Could you check a few things on this model? Use its own coordinates, in mm. A direction names the side the tool comes from. Give positions to 0.01 mm unless a question says otherwise; leave off trailing zeros. Loops run counter-clockwise (first coordinate to the right, second up) from the corner with the lowest first, then second, coordinate; pieces in that order, holes last. Notation, with made-up numbers: M 66.25,21.5 L 102.25,21.5 A19 ccw 102.25,43.5 Z; hole C 24.25,-11.5 d1. An arc over 180 degrees is marked long. Answer in a Markdown table with one row per item. Add a question column.
```python
from build123d import *

# Parameters (mm, degrees)
SKETCH1_R                = 14.5
BOSS_EXTRUDE1_DEPTH      = 11.6
SKETCH2_R                = 11.35
BOSS_EXTRUDE2_DEPTH      = 5
SKETCH3_R                = 4.35
BOSS_EXTRUDE3_DEPTH      = 7
SKETCH4_R                = 2.95
BOSS_EXTRUDE4_DEPTH      = 9
SKETCH5_R                = 2.5
BOSS_EXTRUDE5_DEPTH      = 11.6
SKETCH6_R                = 1.5
BOSS_EXTRUDE6_DEPTH      = 2.8
BOSS_EXTRUDE6_DEPTH_BACK = 16.6


with BuildPart() as part:
    # Sketch1 → Boss-Extrude1 (new body)
    with BuildSketch(Plane(origin=(0, 0, 0), x_dir=(1, 0, 0), z_dir=(0, 1, 0))):
        Circle(SKETCH1_R)
    extrude(amount=BOSS_EXTRUDE1_DEPTH)

    # Sketch2 → Boss-Extrude2 (add)
    with BuildSketch(Plane(origin=(0, 11.6, 0), x_dir=(1, 0, 0), z_dir=(0, 1, 0))):
        Circle(SKETCH2_R)
    extrude(amount=BOSS_EXTRUDE2_DEPTH)

    # Sketch3 → Boss-Extrude3 (add)
    with BuildSketch(Plane(origin=(0, 16.6, 0), x_dir=(1, 0, 0), z_dir=(0, 1, 0))):
        Circle(SKETCH3_R)
    extrude(amount=BOSS_EXTRUDE3_DEPTH)

    # Sketch4 → Boss-Extrude4 (add)
    with BuildSketch(Plane(origin=(0, 23.6, 0), x_dir=(1, 0, 0), z_dir=(0, 1, 0))):
        Circle(SKETCH4_R)
    extrude(amount=BOSS_EXTRUDE4_DEPTH)

    # Sketch5 → Boss-Extrude5 (add)
    with BuildSketch(Plane.XZ):
        with Locations((0, 14.5)):
            Circle(SKETCH5_R)
        with Locations((0, -14.5)):
            Circle(SKETCH5_R)
    extrude(amount=-BOSS_EXTRUDE5_DEPTH)

    # Sketch6 → Boss-Extrude6 (add, two sides)
    with BuildSketch(Plane(origin=(0, 16.6, 0), x_dir=(1, 0, 0), z_dir=(0, 1, 0))) as boss_extrude6_sk:
        with Locations((12.4, 0)):
            Circle(SKETCH6_R)
    extrude(amount=BOSS_EXTRUDE6_DEPTH)
    extrude(boss_extrude6_sk.sketch, amount=-BOSS_EXTRUDE6_DEPTH_BACK)


solid = part.part
```
Item 1: Suppose I cut it at D-D (x = 12.4). List the corners of the cut face in (y, z) for me.
Item 2: For faces 1 (the face through (12, 19.4, 0)), 2 (the face through (-0.943, 20.051, 4.247)), 3 (the face through (14.497, 5.719, 0.284)), which set-ups out of +Z, -Z, +X, -X, +Y, -Y let a thin tool reach every point of the face, with its end or its side?
Item 3: Suppose I cut it at A-A (x = 0). List the corners of the cut face in (y, z) for me.
Item 4: Suppose I cut it at C-C (y = 8). List the corners of the cut face in (x, z) for me.
Item 5: Suppose I cut it at B-B (z = -5.5). List the corners of the cut face in (x, y) for me.
Item 6: I need wall thicknesses on L1, parallel to Y at x = 1.5, z = 13.5; L2, parallel to Y at x = 0.75, z = 5; L3, parallel to Z at x = 5, y = 15. Which ranges of each line are inside material? Lowest first, please.
Item 7: For P1, Ø5, axis at y = 10.5, z = 10.5, coming from the +X side; P2, Ø2.5, axis at x = 11.5, z = 0, coming from the +Y side; P3, Ø1, axis at y = 5.5, z = 11.5, coming from the -X side, each with a flat end and sliding along its axis, tell me the tip position at first contact or that it passes through.
Values found:
| question | item | result |
|---|---|---|
| 1 | outline | M 0,-7.52 L 11.6,-7.52 L 11.6,-1.5 L 19.4,-1.5 L 19.4,1.5 L 11.6,1.5 L 11.6,7.52 L 0,7.52 Z |
| 2 | face 1 | +Z, -Z, +X, +Y |
| 2 | face 2 | +Y |
| 2 | face 3 | +X, +Y, -Y |
| 3 | outline | M 0,-17 L 11.6,-17 L 11.6,-11.35 L 16.6,-11.35 L 16.6,-4.35 L 23.6,-4.35 L 23.6,-2.95 L 32.6,-2.95 L 32.6,2.95 L 23.6,2.95 L 23.6,4.35 L 16.6,4.35 L 16.6,11.35 L 11.6,11.35 L 11.6,17 L 0,17 Z |
| 4 | outline | M -2.49,-14.28 A2.5 ccw long 2.49,-14.28 A14.5 ccw 2.49,14.28 A2.5 ccw long -2.49,14.28 A14.5 ccw Z |
| 5 | outline | M -13.42,0 L 13.42,0 L 13.42,11.6 L 9.93,11.6 L 9.93,16.6 L -9.93,16.6 L -9.93,11.6 L -13.42,11.6 Z |
| 6 | L1 | 0 to 11.6 |
| 6 | L2 | 0 to 16.6 |
| 6 | L3 | -10.19 to 10.19 |
| 7 | P1 | x = 12.09 |
| 7 | P2 | y = 19.4 |
| 7 | P3 | x = -9.45 |
